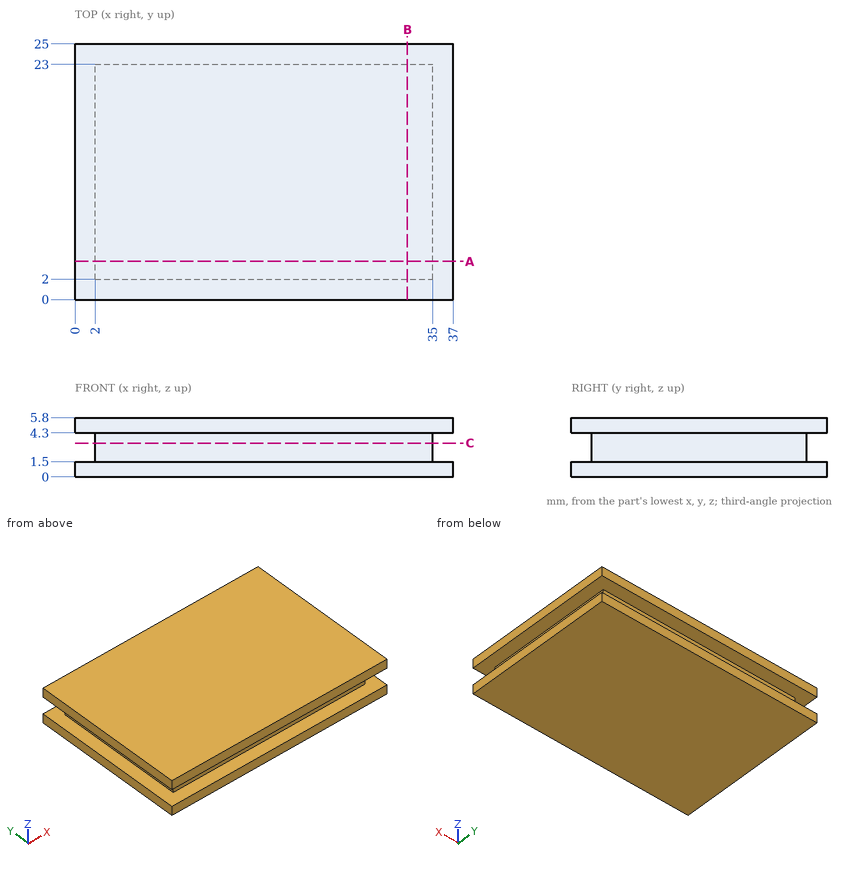
The figure shows three views and two pictorial views of one solid part (mm, origin at its lowest corner). Answer the questions. Round coordinates to 2 decimals unless told otherwise and drop trailing zeros. Write each loop counter-clockwise with the first axis right and the second up, starting at its lowest first coordinate (ties: lowest second). Pieces come first, ordered by that corner, then holes. Notation, with made-up numbers: (23.5, 40) - (80.5, 40) arc R22 cw to (80.5, 47) - close; hole circle Ø3 at (64, 3). An arc over 180 degrees is marked (long way). Use one line per item in the form item = value. Start each with the question number.
Item 1: A cutting plane is placed at C-C (z = 3.3). Write down the section's boundary in (x, y), plus the area to 3 significant figures.
Item 2: A cutting plane is placed at B-B (x = 32.5). Write down the section's boundary in (y, z).
Item 3: Find the intervals of material crossed by line 1 (Y direction, x = 17, z = 2.3); line 2 (X direction, y = 3.75, z = 2.7), in increasing order. Write a range as [from, to].
Item 4: A cutting plane is placed at A-A (y = 3.75). Write down the section's boundary in (x, z), plus the area to 3 significant figures.
Item 5: Flat-ended cylindrical pins translate along their axes: pin 1 Ø0.8 at (y, z) = (12, 3) entering from -X; pin 2 Ø1.4 at (x, z) = (11, 2.5) entering from -Y. Find the tip coordinate at first contact, or state that the pin passes through.
The answers:
q1.outline = (2, 2) - (35, 2) - (35, 23) - (2, 23) - close
q1.area = 693 mm^2
q2.outline = (0, 0) - (25, 0) - (25, 1.5) - (23, 1.5) - (23, 4.3) - (25, 4.3) - (25, 5.8) - (0, 5.8) - (0, 4.3) - (2, 4.3) - (2, 1.5) - (0, 1.5) - close
q3.line_1 = [2, 23]
q3.line_2 = [2, 35]
q4.outline = (0, 0) - (37, 0) - (37, 1.5) - (35, 1.5) - (35, 4.3) - (37, 4.3) - (37, 5.8) - (0, 5.8) - (0, 4.3) - (2, 4.3) - (2, 1.5) - (0, 1.5) - close
q4.area = 203 mm^2
q5.pin_1 = 2
q5.pin_2 = 2
